Design review of the part built by this model. Coordinates are the model's own, in mm. A direction names the side the tool comes from. Round coordinates to 2 decimals unless told otherwise and drop trailing zeros. Loops run counter-clockwise (first coordinate to the right, second up) from the corner with the lowest first, then second, coordinate; pieces in that order, holes last. Notation, with made-up numbers: (70.25, -26.5) -> (125.25, -26.5) arc R19 cw to (125.25, -6.5) -> close; hole circle Ø5 at (68.5, -14). An arc over 180 degrees is marked (long way). Answer as CSV lines item,"result". Start each with the question number.
```python
from build123d import *

# Parameters (mm, degrees)
F1_DEPTH = 25.4
F2_W     = 21.8606553972
F2_H     = 22.4436074495
F3_DEPTH = 12.446
F4_R     = 3.7327062706
F4_R_2   = 3.6053518758
F5_DEPTH = 25.4


# Not quite as in the source:
# - ends of sketch curves that miss each other by under 0.0002 mm in the source are joined


with BuildPart() as f1:
    # F0 (on Front) → F1 (new body)
    with BuildSketch(Plane.XZ):
        Polygon((25.2813665716, 30.7506565005), (-8.463e-07, 30.7506565005), (-8.463e-07, 0), (50.4252426326, 0), (50.4252426326, 15.3024597093), (34.0256324557, 15.3024597093), align=None)
        Polygon((-8.463e-07, 0), (-8.463e-07, 30.7506565005), (-25.2813665716, 30.7506565005), (-34.0256324557, 15.3024597093), (-50.4252426326, 15.3024597093), (-50.4252426326, 0), align=None)
    extrude(amount=F1_DEPTH)

    # F2 (on face) → F3 (cut)
    with BuildSketch(Plane.XZ.offset(25.4)):
        with Locations((0.4372131079, 20.6947550178)):
            Rectangle(F2_W, F2_H)
    extrude(amount=-F3_DEPTH, mode=Mode.SUBTRACT)

    # F4 (on face) → F5 (cut)
    with BuildSketch(Plane.XY.offset(15.3024597093)):
        with Locations((-42.8468845785, -13.5536063462)):
            Circle(F4_R)
        with Locations((42.8468845785, -13.2621303201)):
            Circle(F4_R_2)
    extrude(amount=-F5_DEPTH, mode=Mode.SUBTRACT)


solid = f1.part
```
Q1. Add section C-C, the plane y = -4.75. Give the boundary of the cut face in (x, z), and give its area (3 significant figures).
Q2. Machinability: for faces 1 (the flat face through (-42.1, -9.7, 15.302)), 2 (the flat face through (40.5, -9.7, 15.302)), 3 (the flat face through (-1, -13, 0)), 4 (the flat face through (50.425, -13, 8)), 5 (the flat face through (-10.493, -19, 20)), which of the approach directions +Z, -Z, +X, -X, +Y, -Y give a long, thin tool a straight path to every point of the face, cutting with its end or side? Answer none if there is none.
Q3. Mouldability with a two-part tool opening along X and no side actions: class faces 6 (the cylindrical face through (39.245, -13.104, 7.758)), 7 (the flat face through (-1, -25.4, 9)), 8 (the flat face through (-50.425, -13, 8)) as pulls with the +X half, pulls with the -X half, needs draft (parallel to the pull), parting line crosses it, or undercut.
Q4. For pin 1 Ø8 at (y, z) = (-5, 24) entering from +X; pin 2 Ø10 at (y, z) = (-22, 22.5) entering from -X; pin 3 Ø13 at (x, y) = (-44.5, -15) entering from +Z; pin 4 Ø6.5 at (x, y) = (42.85, -13.26) entering from +Z, all flat-tipped, find the tip position at first contact; note any pin that passes through.
Q5. Add section D-D, the plane z = 19. Give the boundary of the cut face in (x, y).
Q6. Add section B-B, the plane x = -42. Give the boundary of the cut face in (y, z), and give its area (3 significant figures).
Q7. Add section A-A, the plane y = -11. Give the boundary of the cut face in (x, z), and give its area (3 significant figures).
Q8. To check wall thickness, follow probe 1 along X at (y, z) = (-14, 13); probe 2 along Z at (x, y) = (39, -5.25); probe 3 along Y at (x, z) = (-0.5, 12). State the ranges of each line that lie inside material, in increasing order. Write a range as from..to.
Worked answers:
1,outline,"(-50.43, 0) -> (50.43, 0) -> (50.43, 15.3) -> (34.03, 15.3) -> (25.28, 30.75) -> (-25.28, 30.75) -> (-34.03, 15.3) -> (-50.43, 15.3) -> close"
1,area,"2,460 mm^2"
2,face 1,"+Z, -X, +Y, -Y"
2,face 2,"+Z, +X, +Y, -Y"
2,face 3,"-Z, +X, -X, +Y, -Y"
2,face 4,"+Z, -Z, +X, +Y, -Y"
2,face 5,"+Z, -Y"
3,face 6,"undercut"
3,face 7,"needs draft"
3,face 8,"pulls with the -X half"
4,pin 1,"stops at x = 31.37"
4,pin 2,"stops at x = -32.78"
4,pin 3,"stops at z = 15.3"
4,pin 4,"passes through"
5,outline,"(-31.93, -25.4) -> (-10.49, -25.4) -> (-10.49, -12.95) -> (11.37, -12.95) -> (11.37, -25.4) -> (31.93, -25.4) -> (31.93, 0) -> (-31.93, 0) -> close"
6,outline,"(-25.4, 0) -> (-17.19, 0) -> (-17.19, 15.3) -> (-25.4, 15.3) -> close; (-9.92, 0) -> (0, 0) -> (0, 15.3) -> (-9.92, 15.3) -> close"
6,area,"277 mm^2"
7,outline,"(-50.43, 0) -> (-45.57, 0) -> (-45.57, 15.3) -> (-50.43, 15.3) -> close; (-40.12, 0) -> (40.04, 0) -> (40.04, 15.3) -> (34.03, 15.3) -> (25.28, 30.75) -> (-25.28, 30.75) -> (-34.03, 15.3) -> (-40.12, 15.3) -> close; (45.65, 0) -> (50.43, 0) -> (50.43, 15.3) -> (45.65, 15.3) -> close"
7,area,"2,290 mm^2"
8,probe 1,"x = -50.43..-46.55, -39.14..-10.49, 11.37..39.32, 46.38..50.43"
8,probe 2,"z = 0..15.3"
8,probe 3,"y = -12.95..0"
